Model file for the job. Use its own axes, mm. A direction names the side the tool comes from. Round coordinates to 2 decimals unless told otherwise and drop trailing zeros. Loops run counter-clockwise (first coordinate to the right, second up) from the corner with the lowest first, then second, coordinate; pieces in that order, holes last.
from build123d import *

# Parameters (mm, degrees)
F1_DEPTH  = 65.786
F2_R      = 4.1764569431
F2_R_2    = 4.4090075628
F3_DEPTH  = 25.4
F2_R_3    = 5.0559602499
F2_R_4    = 3.7416125294
F4_DEPTH  = 25.4
F5_R      = 14.3858151817
F6_DEPTH  = 68.072
F5_R_2    = 22.255871479
F7_DEPTH  = 61.976
F8_R      = 5.08
F9_R      = 25.9662767353
F10_DEPTH = 113.792


# Not quite as in the source:
# - a feature names something its author has since deleted; it is built from what else it names


with BuildPart() as f1:
    # F0 (on Front) → F1 (new body)
    with BuildSketch(Plane.XZ):
        with BuildLine():
            ThreePointArc((-25.7879418184, 0), (0, 25.7879418184), (25.7879418184, 0))
            Line((25.7879418184, 0), (76.1246234179, 0))
            Line((76.1246234179, 0), (76.1246234179, 15.6854130328))
            Line((76.1246234179, 15.6854130328), (47.4599736899, 15.6854130328))
            ThreePointArc((47.4599736899, 15.6854130328), (44.0974699454, 16.6487565032), (41.7552011698, 19.2464937988))
            ThreePointArc((41.7552011698, 19.2464937988), (0.2284915035, 45.2565071244), (-41.4557046581, 19.4996400932))
            ThreePointArc((-41.4557046581, 19.4996400932), (-43.7973018606, 16.9263567372), (-47.1434027, 15.9732177854))
            Line((-47.1434027, 15.9732177854), (-75.83681494, 15.9732177854))
            Line((-75.83681494, 15.9732177854), (-75.83681494, 0))
            Line((-75.83681494, 0), (-25.7879418184, 0))
        make_face()
    extrude(amount=F1_DEPTH)

    # F2 (on face) → F3 (cut)
    with BuildSketch(Plane.XY.offset(15.9732177854)):
        with Locations((-70.1924338937, -7.3858876713)):
            Circle(F2_R)
        with Locations((-69.1219046712, -57.112660259)):
            Circle(F2_R_2)
    extrude(amount=-F3_DEPTH, mode=Mode.SUBTRACT)

    # F2 (on face) → F4 (cut)
    with BuildSketch(Plane.XY.offset(15.9732177854)):
        with Locations((68.7799453735, -7.4367355555)):
            Circle(F2_R_3)
        with Locations((69.0292343497, -57.3799200356)):
            Circle(F2_R_4)
    extrude(amount=-F4_DEPTH, mode=Mode.SUBTRACT)

    # F5 (on Top) → F6 (cut)
    with BuildSketch(Plane.XY):
        with Locations((0, -31.3370935619)):
            Circle(F5_R)
    extrude(amount=F6_DEPTH, mode=Mode.SUBTRACT)

    # F5 (on Top) → F7 (join)
    with BuildSketch(Plane.XY):
        with Locations((0, -31.3370935619)):
            Circle(F5_R_2)
        with Locations((0, -31.3370935619)):
            Circle(F5_R, mode=Mode.SUBTRACT)
    extrude(amount=F7_DEPTH)

    # F8
    f8_edges = [f1.edges().sort_by_distance(p)[0] for p in [
        (76.124623, -65.786, 7.842707),
        (76.124623, 0, 7.842707),
        (-75.836815, 0, 7.986609),
        (-75.836815, -65.786, 7.986609),
    ]]
    fillet(f8_edges, radius=F8_R)

    # F9 (on Front) → F10 (cut)
    with BuildSketch(Plane.XZ):
        Circle(F9_R)
    extrude(amount=F10_DEPTH, mode=Mode.SUBTRACT)


solid = f1.part
Q1. Flat gauge pins, fed straight in: P1, Ø11.5, axis at x = 68.78, y = -7.44, coming from the +Z side; P2, Ø8.5, axis at x = 69.03, y = -57.38, coming from the -Z side; P3, Ø14, axis at x = -69.12, y = -57.11, coming from the +Z side; P4, Ø10, axis at y = -32, z = 48, coming from the -X side. Where does each tip first touch, or does it go through?
Q2. Slice it at C-C on z = 55. Give the cut face in (x, y), plus the area to 3 significant figures.
Q3. Probe line 1 (X direction, y = -4, z = 9.5); line 2 (X direction, y = -25, z = 9.5); line 3 (Y direction, x = 11.5, z = 29). List the from-to ranges inside material, lowest first.
Q4. Slice it at D-D on x = -55.5. Give the cut face in (y, z).
Q5. Slice it at B-B on x = -12. Give the cut face in (y, z).
Q6. Pull direction Y, two halves, no side cores. Call faces 4 (the face through (-74.365, -7.202, 8.098)), 5 (the face through (-75.837, -33, 8)), 6 (the face through (73.602, -5.918, 7.953)), 7 (the face through (20.56, -39.86, 53.09)): pulls with the +Y half, pulls with the -Y half, needs draft (parallel to the pull), parting line crosses it, or undercut.
Q7. Slice it at A-A on z = 12. Give the cut face in (x, y), plus the area to 3 significant figures.
Q8. Tool access for faces 1 (the face through (-61, -32, 15.973)), 2 (the face through (51, -32, 0)), 3 (the face through (62, -32, 15.685)): list every direction of +Z, -Z, +X, -X, +Y, -Y with a clear straight run to the whole face (end or side of a thin tool).
Reply:
1. P1: stops at z = 15.69
1. P2: stops at z = 0
1. P3: stops at z = 15.97
1. P4: stops at x = -22.26
2. outline: circle Ø44.51 at (0, -31.34); hole circle Ø28.77 at (0, -31.34)
2. area: 906 mm2
3. line 1: x = -75.72 to -72.64, -67.75 to -24.17, 24.17 to 65.07, 72.49 to 76.01
3. line 2: x = -75.84 to -24.17, 24.17 to 76.12
3. line 3: y = -65.79 to -39.98, -22.69 to 0
4. outline: (-65.79, 0) - (0, 0) - (0, 15.97) - (-65.79, 15.97) - close
5. outline: (-65.79, 23.03) - (-39.27, 23.03) - (-39.27, 61.98) - (-50.08, 61.98) - (-50.08, 43.65) - (-65.79, 43.65) - close; (-23.4, 23.03) - (0, 23.03) - (0, 43.65) - (-12.59, 43.65) - (-12.59, 61.98) - (-23.4, 61.98) - close
6. face 4: undercut
6. face 5: needs draft
6. face 6: undercut
6. face 7: parting line crosses it
7. outline: (-75.84, -60.71) arc R5.08 ccw to (-70.76, -65.79) - (-23.03, -65.79) - (-23.03, 0) - (-70.76, 0) arc R5.08 ccw to (-75.84, -5.08) - close; (23.03, -65.79) - (71.04, -65.79) arc R5.08 ccw to (76.12, -60.71) - (76.12, -5.08) arc R5.08 ccw to (71.04, 0) - (23.03, 0) - close; hole circle Ø8.35 at (-70.19, -7.39); hole circle Ø8.82 at (-69.12, -57.11); hole circle Ø10.11 at (68.78, -7.44); hole circle Ø7.48 at (69.03, -57.38)
7. area: 6,700 mm2
8. face 1: +Z, -X, +Y, -Y
8. face 2: -Z, +X, -X, +Y, -Y
8. face 3: +Z, +X, +Y, -Y
